Read the model definition and answer for the solid it produces. Units are mm, in the model's axes. Face numbers are marked on the shaded views. Coordinates: 2 decimals unless noted, no trailing zeros. Loops run counter-clockwise (first coordinate to the right, second up) from the corner with the lowest first, then second, coordinate; pieces in that order, holes last. Notation, with made-up numbers: M 19,69 L 65,69 A27 ccw 65,95 Z; hole C -5,-3.5 d7. An arc over 180 degrees is marked long. One line per item, written item: value. Start each with the question number.
1. The part is cut by section C-C (z = 10.25). Write down the section's boundary in (x, y), then the cut area to 3 significant figures.
2. Consider probe 1 along X at (y, z) = (0, 7); probe 2 along Z at (x, y) = (-26.5, 5); probe 3 along X at (y, z) = (14.5, 5.5). Determine where each line is inside the solid, lowest interval first.
3. Flat-ended cylindrical pins translate along their axes: pin 1 (1.5 mm diameter, centred on x = 37, z = 9, fed in from +Y); pin 2 (1.5 mm diameter, centred on y = -42.5, z = 3.5, fed in from +X); pin 3 (8 mm diameter, centred on x = -9.5, y = -0.5, fed in from -Z); pin 4 (1 mm diameter, centred on x = -27, z = 4.5, fed in from -Y). Find the tip coordinate at first contact, or state that the pin passes through.
4. Determine the mould class of the marked faces 1, 2, 3 and 4 for opening direction X: +X half, -X half, draft (parallel to the pull), parting line (faces both ways), or undercut.
5. The part is cut by section A-A (x = 0). Write down the section's boundary in (y, z), then the cut area to 3 significant figures.
```python
from build123d import *

# Parameters (mm, degrees)
SKETCH_R         = 53
PAD_DEPTH        = 2.7
SKETCH001_W      = 3
SKETCH001_H      = 15
REVOLUTION_ANGLE = 360
FILLET_R         = 2
FILLET001_R      = 2


with BuildPart() as part:
    # Sketch → Pad (new body)
    with BuildSketch(Plane.XY):
        Circle(SKETCH_R)
    extrude(amount=PAD_DEPTH)

    # Sketch001 → Revolution (revolve, symmetric)
    with BuildSketch(Plane(origin=(0, 50.25, 0), x_dir=(0, 1, 0), z_dir=(1, 0, 0))) as revolution_sk:
        with Locations((1.5, 7.5)):
            Rectangle(SKETCH001_W, SKETCH001_H)
    revolve(axis=Axis((0, 0, 0), (0, 0, 1)), revolution_arc=REVOLUTION_ANGLE / 2)
    revolve(revolution_sk.sketch, axis=Axis((0, 0, 0), (0, 0, -1)), revolution_arc=REVOLUTION_ANGLE / 2)

    # Fillet
    fillet_edges = [part.edges().sort_by_distance(p)[0] for p in [
        (0, 53.25, 0),
    ]]
    fillet(fillet_edges, radius=FILLET_R)

    # Fillet001
    fillet001_edges = [part.edges().sort_by_distance(p)[0] for p in [
        (0, 50.25, 15),
    ]]
    fillet(fillet001_edges, radius=FILLET001_R)


solid = part.part
```
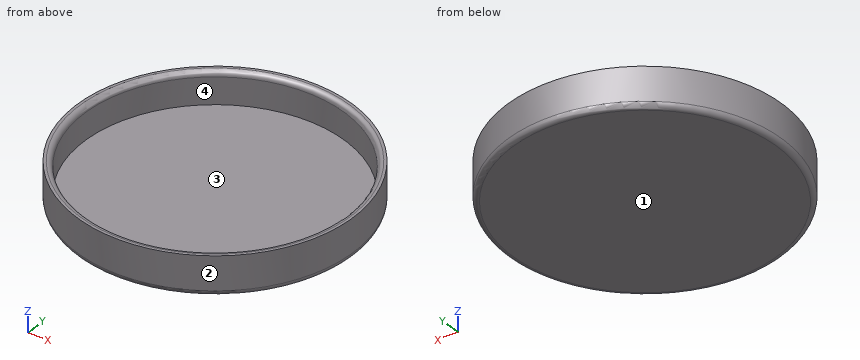
Answer block:
1. outline: C 0,0 d106.5; hole C 0,0 d100.5
1. area: 975 mm2
2. probe 1: x = -53.25 to -50.25, 50.25 to 53.25
2. probe 2: z = 0 to 2.7
2. probe 3: x = -51.24 to -48.11, 48.11 to 51.24
3. pin 1: stops at y = 39.01
3. pin 2: stops at x = 33.05
3. pin 3: stops at z = 0
3. pin 4: stops at y = -46.19
4. face 1: draft
4. face 2: parting line
4. face 3: undercut
4. face 4: undercut
5. outline: M -53.25,2 A2 ccw -51.25,0 L 51.25,0 A2 ccw 53.25,2 L 53.25,15 L 52.25,15 A2 ccw 50.25,13 L 50.25,2.7 L -50.25,2.7 L -50.25,13 A2 ccw -52.25,15 L -53.25,15 Z
5. area: 358 mm2
